from build123d import *


with BuildPart() as part:
    # Croquis3 → Revolución1 (revolve)
    with BuildSketch(Plane(origin=(0, 0, 0), x_dir=(0, 0, -1), z_dir=(1, 0, 0)), mode=Mode.PRIVATE) as revoluci_n1_sk:
        Polygon((40, 0), (50, 0), (50, 60), (40, 60), (40, 70), (-40, 70), (-40, 60), (-50, 60), (-50, 30), (-40, 30), (-40, 50), (-30, 50), (-30, 60), (30, 60), (30, 50), (40, 50), align=None)
    revolve(revoluci_n1_sk.sketch.rotate(Axis((0, 0, 147.034921683), (0, 0, -1)), 90), axis=Axis((0, 0, 147.034921683), (0, 0, -1)))


solid = part.part
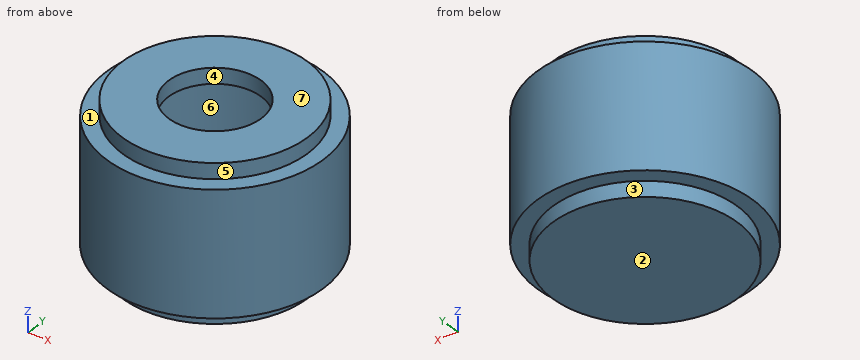
CAD build for the part. Positions are in the model's coordinates, mm. Face numbers are marked on the shaded views. A direction names the side the tool comes from. Round coordinates to 2 decimals unless told otherwise and drop trailing zeros. Loops run counter-clockwise (first coordinate to the right, second up) from the corner with the lowest first, then second, coordinate; pieces in that order, holes last.
(1) Two-plate mould, pull along Y, no slides. Class the marked faces 4, 5, 6 and 7: +Y half, -Y half, draft (parallel to the pull), parting line (faces both ways), or undercut.
(2) Which spindle directions (+Z, -Z, +X, -X, +Y, -Y) get a long thin tool onto all of the face, cutting with end or side? Do the marked faces 1, 2 and 3. Say none if no direction does.
(3) Cut at C-C (y = 46). Give the cut face in (x, z), plus the area to 3 significant figures.
(4) Cut at B-B (z = -37). Give the cut face in (x, y), plus the area to 3 significant figures.
(5) Wall check: line 1 along Z through (x, y) = (-27.5, -51.5); line 2 along X through (y, z) = (1, -14); line 3 along Y through (x, z) = (0, 42.25). Give the ranges that are in metal, low to high.
(6) Drop flat-ended pins along their axis: pin 1 (6 mm diameter, centred on y = 27.5, z = -26, fed in from +X); pin 2 (4 mm diameter, centred on y = -36, z = -17.5, fed in from -X); pin 3 (10 mm diameter, centred on y = -36.5, z = 27.5, fed in from +X). Give the stop position or say it passes through.
(7) Cut at A-A (x = 0). Give the cut face in (y, z), plus the area to 3 significant figures.
Findings below:
1. face 4: undercut
1. face 5: parting line
1. face 6: undercut
1. face 7: draft
2. face 1: +Z
2. face 2: -Z, +X, -X, +Y, -Y
2. face 3: -Z
3. outline: (-52.76, -40) - (-38.52, -40) - (-38.52, -50) - (38.52, -50) - (38.52, -40) - (52.76, -40) - (52.76, 40) - (38.52, 40) - (38.52, 50) - (-38.52, 50) - (-38.52, 40) - (-52.76, 40) - close; hole (-38.52, -30) - (-19.6, -30) - (-19.6, -40) - (19.6, -40) - (19.6, -30) - (38.52, -30) - (38.52, 30) - (19.6, 30) - (19.6, 40) - (-19.6, 40) - (-19.6, 30) - (-38.52, 30) - close
3. area: 4,580 mm2
4. outline: circle Ø140 at (0, 0); hole circle Ø100 at (0, 0)
4. area: 7,540 mm2
5. line 1: z = -50 to -30, 30 to 50
5. line 2: x = -69.99 to -59.99, 59.99 to 69.99
5. line 3: y = -60 to -30, 30 to 60
6. pin 1: stops at x = 65.57
6. pin 2: stops at x = -61.19
6. pin 3: stops at x = 62.51
7. outline: (-70, -40) - (-60, -40) - (-60, -50) - (60, -50) - (60, -40) - (70, -40) - (70, 40) - (60, 40) - (60, 50) - (30, 50) - (30, 40) - (50, 40) - (50, 30) - (60, 30) - (60, -30) - (50, -30) - (50, -40) - (-50, -40) - (-50, -30) - (-60, -30) - (-60, 30) - (-50, 30) - (-50, 40) - (-30, 40) - (-30, 50) - (-60, 50) - (-60, 40) - (-70, 40) - close
7. area: 3,800 mm2
